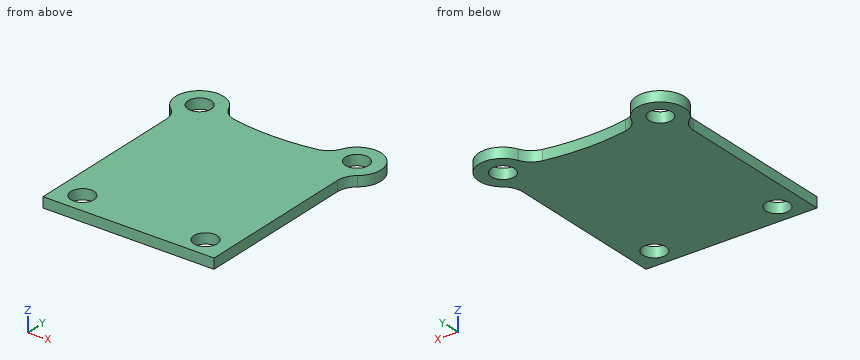
from build123d import *

# Parameters (mm, degrees)
EXTRUDE_1_DEPTH       = 1.5
HOLE_WIZARD_M31_D     = 3.4
HOLE_WIZARD_M31_DEPTH = 1.5


with BuildPart() as part:
    # Эскиз1 → Бобышка-Вытянуть1 (new body)
    with BuildSketch(Plane.XY):
        with BuildLine():
            Line((-12.5, -56.123475383), (-12.5, -80))
            Line((-12.5, -80), (12.5, -80))
            Line((12.5, -80), (12.5, -56.123475383))
            ThreePointArc((12.5, -56.123475383), (12.803848897, -54.807888354), (13.653846154, -53.758794437))
            ThreePointArc((13.653846154, -53.758794437), (13.623122203, -48.217491759), (8.270384407, -49.651080759))
            ThreePointArc((8.270384407, -49.651080759), (7.388025887, -50.827983152), (6.0522893, -51.4439893))
            ThreePointArc((6.0522893, -51.4439893), (0, -52.003676272), (-6.0522893, -51.4439893))
            ThreePointArc((-6.0522893, -51.4439893), (-7.388025887, -50.827983152), (-8.270384407, -49.651080759))
            ThreePointArc((-8.270384407, -49.651080759), (-13.623122203, -48.217491759), (-13.653846154, -53.758794437))
            ThreePointArc((-13.653846154, -53.758794437), (-12.803848897, -54.807888354), (-12.5, -56.123475383))
        make_face()
    extrude(amount=-EXTRUDE_1_DEPTH)

    # Отверстие с зазором M31
    with Locations(Plane.XY):
        with Locations((11.5, -51), (-11.5, -51), (9, -77), (-9, -77)):
            Hole(HOLE_WIZARD_M31_D / 2, depth=HOLE_WIZARD_M31_DEPTH)


solid = part.part
Geometry check sheet. Reference: the model listing, model coordinates, mm. Give positions to 0.01 mm unless a question says otherwise; leave off trailing zeros. Order: outer loops, then holes, each group sorted by start corner. A loop starts at its lowest first (then second) coordinate and runs counter-clockwise, first axis right, second up. Notation, with made-up numbers: M -7.75,3 L 47.25,3 A19 cw 47.25,32 Z; hole C 82,36 d5. An arc over 180 degrees is marked long. Use a Markdown table: item, result.
Item 1: Depth check by flat-ended pin: P1, Ø2, axis at x = 9, y = -77, coming from the -Z side; P2, Ø10, axis at x = 2.5, y = -59.5, coming from the +Z side; P3, Ø0.8, axis at y = -70.5, z = -1, coming from the +X side. Enter the tip coordinate at first touch or a pass-through.
Answers follow:
| item | result |
|---|---|
| P1 | passes through |
| P2 | stops at z = 0 |
| P3 | stops at x = 12.5 |
Item 2: Section check A-A (y = -77). Record the cut outline in (x, z).
Answers follow:
| item | result |
|---|---|
| outline | M -12.5,-1.5 L -10.7,-1.5 L -10.7,0 L -12.5,0 Z; M -7.3,-1.5 L 7.3,-1.5 L 7.3,0 L -7.3,0 Z; M 10.7,-1.5 L 12.5,-1.5 L 12.5,0 L 10.7,0 Z |
Item 3: Section check D-D (y = -51). Record the cut outline in (x, z), and give its area (3 significant figures).
Answers follow:
| item | result |
|---|---|
| outline | M -15,-1.5 L -13.2,-1.5 L -13.2,0 L -15,0 Z; M -9.8,-1.5 L -7.15,-1.5 L -7.15,0 L -9.8,0 Z; M 7.15,-1.5 L 9.8,-1.5 L 9.8,0 L 7.15,0 Z; M 13.2,-1.5 L 15,-1.5 L 15,0 L 13.2,0 Z |
| area | 13.3 mm2 |
Item 4: Section check C-C (z = -0.4). Record the cut outline in (x, y), and give its area (3 significant figures).
Answers follow:
| item | result |
|---|---|
| outline | M -13.65,-53.76 A3 cw -12.5,-56.12 L -12.5,-80 L 12.5,-80 L 12.5,-56.12 A3 cw 13.65,-53.76 A3.5 ccw long 8.27,-49.65 A3 cw 6.05,-51.44 A33 cw -6.05,-51.44 A3 cw -8.27,-49.65 A3.5 ccw long Z; hole C -11.5,-51 d3.4; hole C -9,-77 d3.4; hole C 9,-77 d3.4; hole C 11.5,-51 d3.4 |
| area | 731 mm2 |
Item 5: Material ranges on line 1 along X through (y, z) = (-52.5, -0.2); line 2 along X through (y, z) = (-77, -0.3); line 3 along X through (y, z) = (-50.5, -0.5), recorded low to high.
Answers follow:
| item | result |
|---|---|
| line 1 | x = -14.66 to -12.3, -10.7 to 10.7, 12.3 to 14.66 |
| line 2 | x = -12.5 to -10.7, -7.3 to 7.3, 10.7 to 12.5 |
| line 3 | x = -14.96 to -13.12, -9.88 to -7.73, 7.73 to 9.88, 13.12 to 14.96 |
Item 6: Section check B-B (x = -11.5). Record the cut outline in (y, z).
Answers follow:
| item | result |
|---|---|
| outline | M -80,-1.5 L -52.7,-1.5 L -52.7,0 L -80,0 Z; M -49.3,-1.5 L -47.5,-1.5 L -47.5,0 L -49.3,0 Z |
